Input: dimensioned drawing with shaded views. Units: mm. Origin: part minimum x, y, z. A direction names the side the tool comes from. Coordinates: 2 decimals unless noted, no trailing zeros. Loops run counter-clockwise (first coordinate to the right, second up) from the corner with the lowest first, then second, coordinate; pieces in that order, holes last.
Item 1: Section C-C on z = 17. Return loops of the section in (x, y).
Item 2: Section D-D on x = 43.5. Return loops of the section in (y, z), and give its area (3 significant figures).
Item 3: Contact query for flat-ended pins moving along their axis: P1, Ø3, axis at x = 40.5, z = 12, coming from the +Y side; P2, Ø6, axis at y = 33.5, z = 10, coming from the +X side; P3, Ø8, axis at x = 30.5, z = 9, coming from the -Y side; P4, Ø10, axis at y = 55, z = 18.5, coming from the -X side. Output: stop coordinate, or through.
Item 4: Section A-A on x = 28.5. Return loops of the section in (y, z).
Item 5: Section B-B on y = 75.2. Return loops of the section in (x, z), and give its area (3 significant figures).
Item 6: Ray query, line 1 along Z through (x, y) = (8.5, 55); line 2 along X through (y, z) = (92.5, 16); line 3 along Y through (x, z) = (7.5, 13.25). Return the intervals inside material, ascending.
Item 7: Reachability of the marked faces 1, 2 and 3 from +Z, -Z, +X, -X, +Y, -Y: full face, straight path, thin tool, end or side. Return the list, or none.
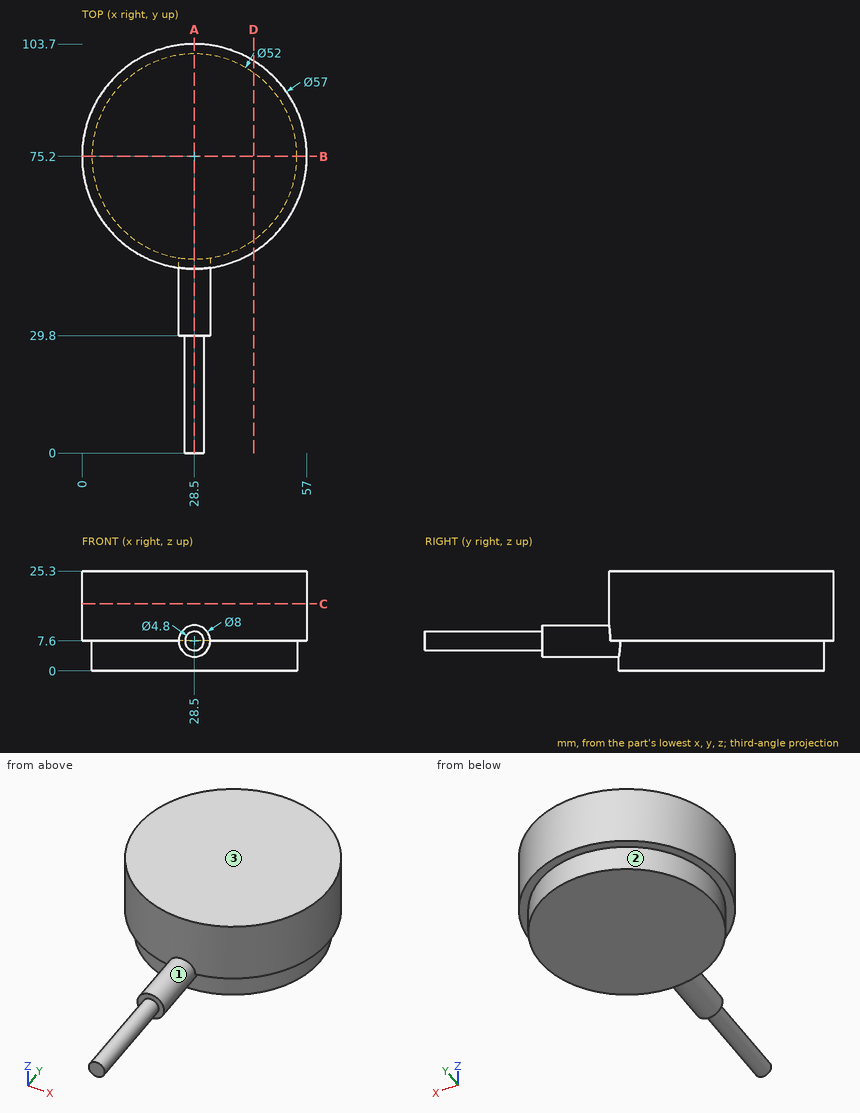
Results found:
1. outline: circle Ø57 at (28.5, 75.2)
2. outline: (50.97, 7.6) - (53.96, 7.6) - (53.96, 0) - (96.44, 0) - (96.44, 7.6) - (99.43, 7.6) - (99.43, 25.3) - (50.97, 25.3) - close
2. area: 1,180 mm2
3. P1: stops at y = 101.7
3. P2: stops at x = 32.5
3. P3: stops at y = 0
3. P4: stops at x = 4.39
4. outline: (0, 5.2) - (29.8, 5.2) - (29.8, 3.6) - (49.2, 3.6) - (49.2, 0) - (101.2, 0) - (101.2, 7.6) - (103.7, 7.6) - (103.7, 25.3) - (46.7, 25.3) - (46.7, 11.6) - (29.8, 11.6) - (29.8, 10) - (0, 10) - close
5. outline: (0, 7.6) - (2.5, 7.6) - (2.5, 0) - (54.5, 0) - (54.5, 7.6) - (57, 7.6) - (57, 25.3) - (0, 25.3) - close
5. area: 1,400 mm2
6. line 1: z = 7.6 to 25.3
6. line 2: x = 5.85 to 51.15
6. line 3: y = 55.93 to 94.47
7. face 1: -Y
7. face 2: -Z
7. face 3: +Z, +X, -X, +Y, -Y
